Work out the finished part from the listing and answer in its coordinate system (mm). Face numbers are marked on the shaded views. A direction names the side the tool comes from. Round coordinates to 2 decimals unless told otherwise and drop trailing zeros. Loops run counter-clockwise (first coordinate to the right, second up) from the corner with the lowest first, then second, coordinate; pieces in that order, holes last. Notation, with made-up numbers: M 10,52.25 L 62,52.25 A23 ccw 62,76.25 Z; hole C -21,13.25 d1. An arc over 180 degrees is marked long. One line per item, written item: value.
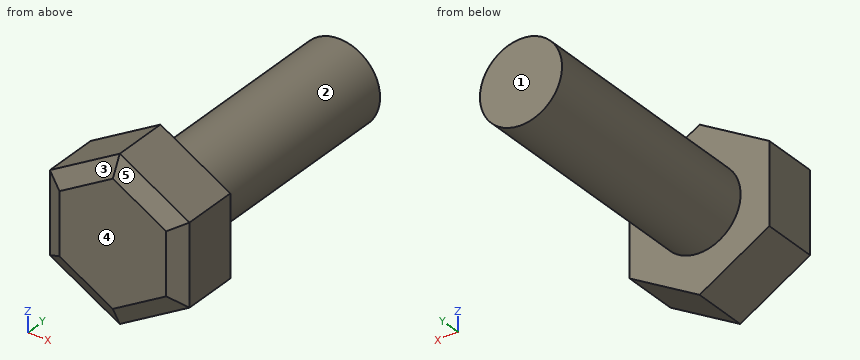
```python
from build123d import *

# Parameters (mm, degrees)
EXTRUDE_1_DEPTH = 8
SKETCH_2_R      = 5
EXTRUDE_2_DEPTH = 30
CHAMFER_1_SIZE  = 2
CHAMFER_1_SIZE2 = 1.154700538


with BuildPart() as part:
    # Эскиз1 → Бобышка-Вытянуть1 (new body)
    with BuildSketch(Plane(origin=(0, 0, 0), x_dir=(1, 0, 0), z_dir=(0, 1, 0))):
        Polygon((8.5, -4.907477288), (8.5, 4.907477288), (0, 9.814954576), (-8.5, 4.907477288), (-8.5, -4.907477288), (0, -9.814954576), align=None)
    extrude(amount=EXTRUDE_1_DEPTH)

    # Эскиз2 → Бобышка-Вытянуть2 (add)
    with BuildSketch(Plane(origin=(0, 8, 0), x_dir=(1, 0, 0), z_dir=(0, 1, 0))):
        Circle(SKETCH_2_R)
    extrude(amount=EXTRUDE_2_DEPTH)

    # Фаска1
    chamfer_1_edges = [part.edges().sort_by_distance(p)[0] for p in [
        (-4.25, 0, 7.361215932),
        (-8.5, 0, 0),
        (-4.25, 0, -7.361215932),
        (4.25, 0, -7.361215932),
        (8.5, 0, 0),
        (4.25, 0, 7.361215932),
    ]]
    chamfer_1_side = [part.faces().sort_by_distance(p)[0] for p in [
        (0, 0, 0),
    ]]
    chamfer(chamfer_1_edges, length=CHAMFER_1_SIZE, length2=CHAMFER_1_SIZE2, reference=chamfer_1_side[0])


solid = part.part
```
1) Find the intervals of material crossed by probe 1 along Y at (x, z) = (-3.5, -3.75); probe 2 along Y at (x, z) = (0.5, 8.25); probe 3 along Z at (x, y) = (-2.5, 20.5), in increasing order. Write a range as from..to.
Check values:
probe 1: 0..8
probe 2: 0.52..8
probe 3: -4.33..4.33
2) The mould has two halves that part along X. Classify the marked faces 3, 4 and 5: +X half, -X half, draft (parallel to the pull), parting line (faces both ways), or undercut.
Check values:
face 3: -X half
face 4: draft
face 5: +X half
3) For the marked faces 1 and 2, determine the directions among +Z, -Z, +X, -X, +Y, -Y from which every point of the face is accessible in a straight line to the end or side of a thin tool.
Check values:
face 1: +Z, -Z, +X, -X, +Y
face 2: +Y
4) Find section A-A (z = 0). Give the vertices of the cut face in (x, y).
Check values:
outline: M -8.5,1.15 L -6.5,0 L 6.5,0 L 8.5,1.15 L 8.5,8 L 5,8 L 5,38 L -5,38 L -5,8 L -8.5,8 Z
5) Find section D-D (z = 8). Give the vertices of the cut face in (x, y).
Check values:
outline: M -3.14,1.15 L 0,0.25 L 3.14,1.15 L 3.14,8 L -3.14,8 Z
6) Find section B-B (y = 33). Give the vertices of the cut face in (x, z), then the cut area to 3 significant figures.
Check values:
outline: C 0,0 d10
area: 78.5 mm2
7) Find section C-C (x = -6). Give the vertices of the cut face in (y, z).
Check values:
outline: M 0,-4.04 L 1.15,-6.35 L 8,-6.35 L 8,6.35 L 1.15,6.35 L 0,4.04 Z
8) Each of these flat-tipped pins is pushed along its axis until it touches: pin 1 (1.5 mm diameter, centred on y = 20, z = 6.5, fed in from -X); pin 2 (1 mm diameter, centred on x = -6.5, z = -1.5, fed in from +Y); pin 3 (8 mm diameter, centred on x = -5, y = 25.5, fed in from +Z); pin 4 (1 mm diameter, centred on y = 12.5, z = -3.5, fed in from +X). Where does it stop, or does it pass through?
Check values:
pin 1: through
pin 2: y = 8
pin 3: z = 4.9
pin 4: x = 4
